Source: CAD feature listing. Evaluate the final solid. Frame: model axes, mm. Face numbers are marked on the shaded views. A direction names the side the tool comes from. Give positions to 0.01 mm unless a question says otherwise; leave off trailing zeros. Order: outer loops, then holes, each group sorted by start corner. A loop starts at its lowest first (then second) coordinate and runs counter-clockwise, first axis right, second up. Notation, with made-up numbers: (4.25, -21.5) - (20.25, -21.5) arc R17 cw to (20.25, 3.5) - close; hole circle Ø8 at (64, 43). An arc over 180 degrees is marked (long way). Answer as CSV lines item,"result".
```python
from build123d import *

# Parameters (mm, degrees)
SKETCH1_W           = 70
SKETCH1_H           = 20
SKETCH1_R           = 4
BOSS_EXTRUDE1_DEPTH = 5
SKETCH2_W           = 15
SKETCH2_H           = 20
BOSS_EXTRUDE2_DEPTH = 6
SKETCH3_R           = 4
CUT_EXTRUDE1_DEPTH  = 46.923850013
FILLET1_R           = 2


with BuildPart() as part:
    # Sketch1 → Boss-Extrude1 (new body)
    with BuildSketch(Plane(origin=(0, 0, 0), x_dir=(1, 0, 0), z_dir=(0, 1, 0))):
        Rectangle(SKETCH1_W, SKETCH1_H)
        with Locations(Location((-25, 0, 0), (0, 0, 270))):
            Circle(SKETCH1_R, mode=Mode.SUBTRACT)
        with Locations(Location((25, 0, 0), (0, 0, 90))):
            Circle(SKETCH1_R, mode=Mode.SUBTRACT)
    boss_extrude1 = extrude(amount=BOSS_EXTRUDE1_DEPTH)

    # Sketch2 → Boss-Extrude2 (add)
    with BuildSketch(Plane(origin=(0, 5, 0), x_dir=(1, 0, 0), z_dir=(0, 1, 0))):
        Rectangle(SKETCH2_W, SKETCH2_H)
    boss_extrude2 = extrude(amount=BOSS_EXTRUDE2_DEPTH)

    # Mirror3: Boss-Extrude2 across plane
    add(boss_extrude2.mirror(Plane.ZX.offset(11)))

    # Mirror4: Boss-Extrude1 across plane
    add(boss_extrude1.mirror(Plane.ZX.offset(11)))

    # Sketch3 → Cut-Extrude1 (cut, through all)
    with BuildSketch(Plane(origin=(0, 0, -10), x_dir=(-1, 0, 0), z_dir=(0, 0, -1))):
        with Locations((0, 11)):
            Circle(SKETCH3_R)
    extrude(amount=-CUT_EXTRUDE1_DEPTH, mode=Mode.SUBTRACT)

    # Fillet1
    fillet1_edges = [part.edges().sort_by_distance(p)[0] for p in [
        (7.5, 11, 10),
        (7.5, 11, -10),
        (-7.5, 11, -10),
        (-7.5, 11, 10),
    ]]
    fillet(fillet1_edges, radius=FILLET1_R)


solid = part.part
```
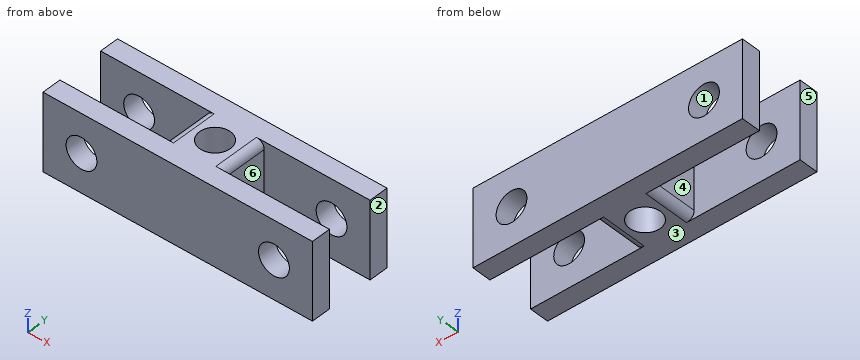
(1) Ray query, line 1 (X direction, y = 18.15, z = 0); line 2 (Z direction, x = 25, y = 18.7); line 3 (Y direction, x = 0, z = -5.5). Return the intervals inside material, ascending. Write a range as from..to.
Completed:
line 1,"-35..-29, -21..21, 29..35"
line 2,"-10..-4, 4..10"
line 3,"0..7, 15..22"
(2) Contact query for flat-ended pins moving along their axis: pin 1 (9.5 mm diameter, centred on y = 10.5, z = -3.5, fed in from +X); pin 2 (1.5 mm diameter, centred on y = 8, z = 7.5, fed in from -X). Output: stop coordinate, or through.
Completed:
pin 1,"x = 7.5"
pin 2,"x = -7.5"
(3) Cut plane A-A (z = 0). Give the number of separate pieces and of enclosed holes in the cut face, then the cut area to 3 significant figures.
Completed:
separate pieces,"5"
enclosed holes,"1"
area,"670 mm²"
(4) Cut plane C-C (y = 11). Return loops of the section in (x, z), then the cut area to 3 significant figures.
Completed:
outline,"(-7.5, -8) arc R2 ccw to (-5.5, -10) - (-4, -10) - (-4, 10) - (-5.5, 10) arc R2 ccw to (-7.5, 8) - close; (4, -10) - (5.5, -10) arc R2 ccw to (7.5, -8) - (7.5, 8) arc R2 ccw to (5.5, 10) - (4, 10) - close"
area,"137 mm²"
(5) Access query for the marked faces 4, 5 and 6. Directions: +Z, -Z, +X, -X, +Y, -Y. A direction counts if a zero-diameter tool reaches every point of the face in a straight line with its end or side. Return the directions, or none.
Completed:
face 4,"+Z, -Z, -X"
face 5,"+Z, -Z, -X, +Y, -Y"
face 6,"+Z, -Z, +X"
(6) Cut plane D-D (x = 0). Return loops of the section in (y, z), then the cut area to 3 significant figures.
Completed:
outline,"(0, -10) - (7, -10) - (7, 10) - (0, 10) - close; (15, -10) - (22, -10) - (22, 10) - (15, 10) - close"
area,"280 mm²"
(7) Mould query, pull axis Z, two halves, no side actions, for the marked faces 1, 2 and 3. Classes: released by +Z, released by -Z, zero draft, split by the parting line, or undercut.
Completed:
face 1,"undercut"
face 2,"zero draft"
face 3,"released by -Z"
(8) Cut plane B-B (x = 25). Return loops of the section in (y, z).
Completed:
outline,"(0, -10) - (5, -10) - (5, -4) - (0, -4) - close; (0, 4) - (5, 4) - (5, 10) - (0, 10) - close; (17, -10) - (22, -10) - (22, -4) - (17, -4) - close; (17, 4) - (22, 4) - (22, 10) - (17, 10) - close"
